Geometry check sheet. Reference: the model listing, model coordinates, mm. Give positions to 0.01 mm unless a question says otherwise; leave off trailing zeros. Loops run counter-clockwise (first coordinate to the right, second up) from the corner with the lowest first, then second, coordinate; pieces in that order, holes last.
1. Cross-section at C-C, the plane z = 0.6. Record the cut outline in (x, y).
2. Cross-section at D-D, the plane x = 28. Record the cut outline in (y, z).
3. Cross-section at A-A, the plane x = 0. Record the cut outline in (y, z).
4. Material ranges on L1, parallel to X at y = 0.5, z = 1.4; L2, parallel to X at y = -30, z = 1.4, recorded low to high.
5. Release check for a two-part mould opening along X. For faces 1 (the flat face through (0, 35, 1)), 2 (the cylindrical face through (31, -9.76, 0.74)), 3 (the flat face through (-35, 0, 1)) record: +X half, -X half, draft (parallel to the pull), parting line (faces both ways), or undercut.
Autodesk Fusion 360 part; units mm, degrees
sketch "Sketch1" plane through (0, 0, 0) normal (0, 0, 1) x (1, 0, 0)
  line L0 (30, -35) -> (-30, -35)
  line L1 (-35, -30) -> (-35, 30)
  line L2 (-30, 35) -> (30, 35)
  line L3 (35, 30) -> (35, -30)
  line L4 (35, -35) -> (-35, 35) construction
  line L5 (-35, -35) -> (35, 35) construction
  circle A0 centre (0, 0) radius 32.5
  circle A1 centre (-28.9896, 28.9896) radius 2.5
  arc A2 (-30, 35) -> (-35, 30) centre (-30, 30) ccw
  arc A3 (35, 30) -> (30, 35) centre (30, 30) ccw
  arc A4 (30, -35) -> (35, -30) centre (30, -30) ccw
  arc A5 (-35, -30) -> (-30, -35) centre (-30, -30) ccw
  line L6 (0, 35) -> (0, -35) construction
  line L7 (-35, 0) -> (35, 0) construction
  circle A6 centre (28.9896, 28.9896) radius 2.5
  circle A7 centre (-28.9896, -28.9896) radius 2.5
  circle A8 centre (28.9896, -28.9896) radius 2.5
  dimension "d1" = 70
  dimension "d2" = 70
  dimension "d3" = 65
  dimension "d4" = 5
  dimension "d5" = 8.5
  dimension "d6" = 5
  dimension "d7" = 5
  dimension "d8" = 5
  dimension "d9" = 5
extrude "Extrude1" add sketch "Sketch1" along normal blind 1.5
Result:
1. outline: (-35, -30) arc R5 ccw to (-30, -35) - (30, -35) arc R5 ccw to (35, -30) - (35, 30) arc R5 ccw to (30, 35) - (-30, 35) arc R5 ccw to (-35, 30) - close; hole circle Ø65 at (0, 0); hole circle Ø5 at (-28.99, -28.99); hole circle Ø5 at (-28.99, 28.99); hole circle Ø5 at (28.99, -28.99); hole circle Ø5 at (28.99, 28.99)
2. outline: (-35, 0) - (-31.29, 0) - (-31.29, 1.5) - (-35, 1.5) - close; (-26.69, 0) - (-16.5, 0) - (-16.5, 1.5) - (-26.69, 1.5) - close; (16.5, 0) - (26.69, 0) - (26.69, 1.5) - (16.5, 1.5) - close; (31.29, 0) - (35, 0) - (35, 1.5) - (31.29, 1.5) - close
3. outline: (-35, 0) - (-32.5, 0) - (-32.5, 1.5) - (-35, 1.5) - close; (32.5, 0) - (35, 0) - (35, 1.5) - (32.5, 1.5) - close
4. L1: x = -35 to -32.5, 32.5 to 35
4. L2: x = -35 to -31.28, -26.7 to -12.5, 12.5 to 26.7, 31.28 to 35
5. face 1: draft
5. face 2: undercut
5. face 3: -X half
